Could you check a few things on this model? Use its own coordinates, in mm. Coordinates: 2 decimals unless noted, no trailing zeros. Order: outer loops, then holes, each group sorted by start corner. A loop starts at its lowest first (then second) coordinate and runs counter-clockwise, first axis right, second up. Notation, with made-up numbers: (82, 28) - (127, 28) arc R11 cw to (127, 44) - close; hole circle Ø2 at (72.25, 62.25). An arc over 180 degrees is marked (long way). One line per item, written item: value.
from build123d import *

# Parameters (mm, degrees)
SKETCH1_W                      = 10
SKETCH1_H                      = 10
BOSS_EXTRUDE1_DEPTH            = 15
F_97_0_0059_DIAMETER_HOLE1_D   = 7.499999986
CUT_EXTRUDE1_DEPTH             = 15
F_0_80_TAPPED_HOLE1_D          = 1.19126
F_0_80_TAPPED_HOLE1_DEPTH      = 4.95
F_0_80_TAPPED_HOLE1_TIP        = 0.357890611
M2X0_4_TAPPED_HOLE1_AT_2_COUNT = 2
M2X0_4_TAPPED_HOLE1_AT_2_PITCH = 8.348802309


with BuildPart() as part:
    # Sketch1 → Boss-Extrude1 (new body)
    with BuildSketch(Plane(origin=(0, 0, 0), x_dir=(1, 0, 0), z_dir=(0, 1, 0))):
        with Locations((5, 5)):
            Rectangle(SKETCH1_W, SKETCH1_H)
    extrude(amount=BOSS_EXTRUDE1_DEPTH)

    # #97 (0.0059) Diameter Hole1 (through all)
    with Locations(Plane(origin=(0, 15, 0), x_dir=(1, 0, 0), z_dir=(0, 1, 0))):
        with Locations((5, 4.5)):
            Hole(F_97_0_0059_DIAMETER_HOLE1_D / 2)

    # Sketch4 → Cut-Extrude1 (cut)
    with BuildSketch(Plane(origin=(10, 0, 0), x_dir=(0, 0, -1), z_dir=(1, 0, 0))):
        Polygon((10, 0), (9, 0), (10, 5.000000002), align=None)
    extrude(amount=-CUT_EXTRUDE1_DEPTH, mode=Mode.SUBTRACT)

    # #0-80 Tapped Hole1
    with Locations(Plane(origin=(0, -1.73076923, -8.653846154), x_dir=(-1, 0, 0), z_dir=(0, -0.19611613506937778, -0.9805806757046814))):
        with Locations((-5, 5.664064731), (-5, 2.864064731)):
            Hole(F_0_80_TAPPED_HOLE1_D / 2, depth=F_0_80_TAPPED_HOLE1_DEPTH)
            with Locations((0, 0, -(F_0_80_TAPPED_HOLE1_DEPTH + F_0_80_TAPPED_HOLE1_TIP / 2))):  # 118° drill point
                Cone(0, F_0_80_TAPPED_HOLE1_D / 2, F_0_80_TAPPED_HOLE1_TIP, mode=Mode.SUBTRACT)

    # Sketch7 → M2x0.4 Tapped Hole1 (revolve, cut)
    with BuildSketch(Plane(origin=(10, 4, -2.3), x_dir=(0, 0, -1), z_dir=(0, 1, 0))):
        Polygon((0, 0), (0, 5.680688495), (0.8, 5.2), (0.8, 0), align=None)
    m2x0_4_tapped_hole1 = revolve(axis=Axis((16.35, 4, -2.3), (-1, 0, 0)), mode=Mode.SUBTRACT)

    # M2x0.4 Tapped Hole1 at 2: M2x0.4 Tapped Hole1 ×2
    with Locations(*[Vector(0, 0.838443616300637, -0.5449883505954144) * (i * M2X0_4_TAPPED_HOLE1_AT_2_PITCH) for i in range(1, M2X0_4_TAPPED_HOLE1_AT_2_COUNT)]):
        add(m2x0_4_tapped_hole1, mode=Mode.SUBTRACT)

    # Mirror1: M2x0.4 Tapped Hole1 across plane
    add(m2x0_4_tapped_hole1.mirror(Plane(origin=(5, 0, 0), x_dir=(0, 0, 1), z_dir=(1, 0, 0))), mode=Mode.SUBTRACT)

    # Mirror1 copy 1 sketch → Mirror1 copy 1 (revolve, cut)
    with BuildSketch(Plane(origin=(0, 11, -6.85), x_dir=(0, 0, -1), z_dir=(0, 1, 0))):
        Polygon((0, 0), (0, -5.680688495), (0.8, -5.2), (0.8, 0), align=None)
    revolve(axis=Axis((-6.35, 11, -6.85), (-1, 0, 0)), mode=Mode.SUBTRACT)


solid = part.part
Item 1: Thinking about a two-plate mould opening in Z: for faces 1 (the face through (4.92, 4.57, -9.05)), 2 (the face through (1.132, 10.76, -7.613)), 3 (the face through (5, 7, 0)), 4 (the face through (3, 0, -8)), which applies, pulls with the +Z half, pulls with the -Z half, needs draft (parallel to the pull), parting line crosses it, or undercut?
Conclusion:
face 1: undercut
face 2: undercut
face 3: pulls with the +Z half
face 4: needs draft
Item 2: I want a section at B-B on z = -2.3. Please give me the cut outline in (x, y).
Conclusion:
outline: (0, 0) - (1.96, 0) - (1.96, 3.2) - (0, 3.2) - close; (0, 4.8) - (1.96, 4.8) - (1.96, 15) - (0, 15) - close; (8.04, 0) - (10, 0) - (10, 3.2) - (8.04, 3.2) - close; (8.04, 4.8) - (10, 4.8) - (10, 15) - (8.04, 15) - close
Item 3: If I drill on probe 1 along Y at (x, z) = (8.1, -6.85); probe 2 along Z at (x, y) = (1.75, 14.25); probe 3 along Y at (x, z) = (0.9, -2.3), over which ranges is the centre line in solid material (lowest first)?
Conclusion:
probe 1: 0 to 10.2, 11.8 to 15
probe 2: -10 to -6.37, -2.63 to 0
probe 3: 0 to 3.2, 4.8 to 15
Item 4: I want a section at C-C on y = 11. Please give me the cut outline in (x, z).
Conclusion:
outline: (0, -10) - (10, -10) - (10, -7.65) - (7.03, -7.65) arc R3.75 cw to (2.97, -7.65) - (0, -7.65) - close; (0, -6.05) - (1.59, -6.05) arc R3.75 cw (long way) to (8.41, -6.05) - (10, -6.05) - (10, 0) - (0, 0) - close
Item 5: I want a section at A-A on z = -4.5. Please give me the cut outline in (x, y), then the cut area to 3 significant figures.
Conclusion:
outline: (0, 0) - (1.25, 0) - (1.25, 15) - (0, 15) - close; (8.75, 0) - (10, 0) - (10, 15) - (8.75, 15) - close
area: 37.5 mm²
Item 6: I'm going to push a flat-ended pin straight in: pin 1 Ø1 at (x, z) = (4, -3) entering from +Y. Where does the tip first touch, or does it pass through?
Conclusion:
pin 1: through
Item 7: I want a section at D-D on x = 3.25. Please give me the cut outline in (y, z).
Conclusion:
outline: (0, -9) - (5, -10) - (15, -10) - (15, -7.82) - (0, -7.82) - close; (0, -1.18) - (15, -1.18) - (15, 0) - (0, 0) - close
